For this review, take the finished solid that the model builds, in its own axes (mm). Face numbers are marked on the shaded views. Give positions to 0.01 mm unless a question says otherwise; leave off trailing zeros. Order: outer loops, then holes, each group sorted by start corner. A loop starts at its lowest first (then second) coordinate and runs counter-clockwise, first axis right, second up.
from build123d import *

# Parameters (mm, degrees)
ESQUISSE1_R        = 5.5
BOSS_EXTRU_1_DEPTH = 5
ESQUISSE3_W        = 10
ESQUISSE3_H        = 54.25
ESQUISSE3_H_2      = 42.75
ESQUISSE3_W_2      = 33
ESQUISSE3_H_3      = 10
BOSS_EXTRU_3_DEPTH = 6
D_POUILLE2_ANGLE   = 10
BOSS_EXTRU_4_DEPTH = 10
CHANFREIN1_SIZE    = 5


with BuildPart() as part:
    # Esquisse1 → Boss.-Extru.1 (new body)
    with BuildSketch(Plane.XY):
        Polygon((-22.5, 135.232443508), (22.5, 135.232443508), (70, -9.767556492), (70, -54.767556492), (-70, -54.767556492), (-70, -9.767556492), align=None)
        with Locations((0, 120.232443508)):
            Circle(ESQUISSE1_R, mode=Mode.SUBTRACT)
        with Locations((0, 43.982443508)):
            Circle(ESQUISSE1_R, mode=Mode.SUBTRACT)
        with Locations((0, -32.267556492)):
            Circle(ESQUISSE1_R, mode=Mode.SUBTRACT)
        with Locations((-55, -32.267556492)):
            Circle(ESQUISSE1_R, mode=Mode.SUBTRACT)
        with Locations((55, -32.267556492)):
            Circle(ESQUISSE1_R, mode=Mode.SUBTRACT)
    extrude(amount=BOSS_EXTRU_1_DEPTH)

    # Esquisse3 → Boss.-Extru.3 (add)
    with BuildSketch(Plane.XY.offset(5)):
        with Locations((0, 82.107443508)):
            Rectangle(ESQUISSE3_W, ESQUISSE3_H)
        with Locations((0, 11.607443508)):
            Rectangle(ESQUISSE3_W, ESQUISSE3_H_2)
        with Locations((-27.5, -32.267556492)):
            Rectangle(ESQUISSE3_W_2, ESQUISSE3_H_3)
        with Locations((27.5, -32.267556492)):
            Rectangle(ESQUISSE3_W_2, ESQUISSE3_H_3)
    extrude(amount=BOSS_EXTRU_3_DEPTH)

    # Dépouille2
    d_pouille2_faces = [part.faces().sort_by_distance(p)[0] for p in [
        (0, 32.982443508, 8),
        (-27.5, -27.267556492, 8),
        (27.5, -27.267556492, 8),
        (0, 109.232443508, 8),
        (-11, -32.267556492, 8),
        (44, -32.267556492, 8),
        (5, 82.107443508, 8),
        (5, 11.607443508, 8),
        (-5, 82.107443508, 8),
        (0, 54.982443508, 8),
        (-5, 11.607443508, 8),
        (11, -32.267556492, 8),
        (27.5, -37.267556492, 8),
        (0, -9.767556492, 8),
        (-44, -32.267556492, 8),
        (-27.5, -37.267556492, 8),
    ]]
    draft(d_pouille2_faces, Plane.XY.offset(5), D_POUILLE2_ANGLE)

    # Esquisse4 → Boss.-Extru.4 (add)
    with BuildSketch(Plane.XY.offset(5)):
        Polygon((-22.75, 134.469285613), (-22.75, -9.517556492), (-69.918103448, -9.517556492), align=None)
        Polygon((22.75, -9.517556492), (69.918103448, -9.517556492), (22.75, 134.469285613), align=None)
    extrude(amount=BOSS_EXTRU_4_DEPTH)

    # Chanfrein1
    chanfrein1_edges = [part.edges().sort_by_distance(p)[0] for p in [
        (-22.75, -9.517556492, 10),
        (22.75, -9.517556492, 10),
    ]]
    chamfer(chanfrein1_edges, length=CHANFREIN1_SIZE)


solid = part.part
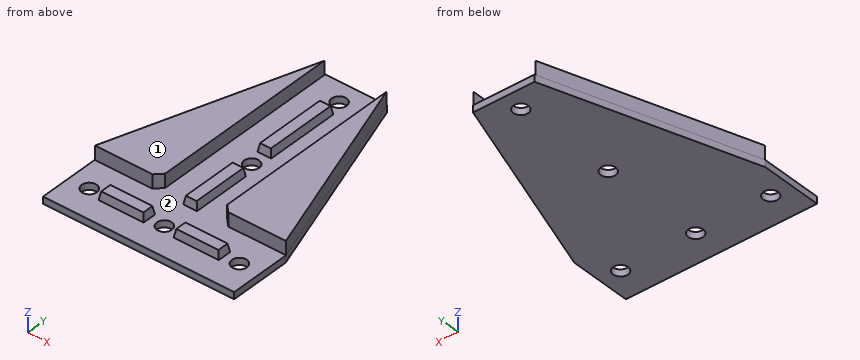
1) Draft analysis for pull direction X (two halves, no side actions). For the marked faces 1 and 2, state which applies: +X half, -X half, draft (parallel to the pull), parting line (faces both ways), or undercut.
Answer sheet:
face 1: draft
face 2: undercut
2) To check wall thickness, follow line 1 (Y direction, x = 0, z = 1.3); line 2 (X direction, y = 6, z = 6.5); line 3 (X direction, y = 80, z = 10). State the ranges of each line that lie inside material, in increasing order.
Answer sheet:
line 1: y = -54.77 to -37.77, -26.77 to 38.48, 49.48 to 114.73, 125.73 to 135.23
line 2: x = -64.83 to -22.75, -4.74 to 4.74, 22.75 to 64.83
line 3: x = -40.59 to -22.75, -4.12 to 4.12, 22.75 to 40.59
3) We need section A-A on x = 0. Give the boundary of the cut face in (y, z), then the cut area to 3 significant figures.
Answer sheet:
outline: (-54.77, 0) - (-37.77, 0) - (-37.77, 5) - (-54.77, 5) - close; (-26.77, 0) - (38.48, 0) - (38.48, 5) - (32.98, 5) - (31.92, 11) - (-8.71, 11) - (-9.77, 5) - (-26.77, 5) - close; (49.48, 0) - (114.73, 0) - (114.73, 5) - (109.23, 5) - (108.17, 11) - (56.04, 11) - (54.98, 5) - (49.48, 5) - close; (125.73, 0) - (135.23, 0) - (135.23, 5) - (125.73, 5) - close
area: 1,350 mm2
4) We need section C-C on y = 12. Give the boundary of the cut face in (x, z), then the cut area to 3 significant figures.
Answer sheet:
outline: (-62.87, 0) - (62.87, 0) - (62.87, 15) - (22.75, 15) - (22.75, 5) - (5, 5) - (3.94, 11) - (-3.94, 11) - (-5, 5) - (-22.75, 5) - (-22.75, 15) - (-62.87, 15) - close
area: 1,480 mm2
5) We need section B-B on x = -55. Give the boundary of the cut face in (y, z).
Answer sheet:
outline: (-54.77, 0) - (-37.77, 0) - (-37.77, 5) - (-54.77, 5) - close; (-26.77, 0) - (36.02, 0) - (36.02, 15) - (-9.52, 15) - (-9.52, 5) - (-26.77, 5) - close
6) We need section D-D on x = 18.5. Give the boundary of the cut face in (y, z).
Answer sheet:
outline: (-54.77, 0) - (135.23, 0) - (135.23, 5) - (-27.27, 5) - (-28.33, 11) - (-36.21, 11) - (-37.27, 5) - (-54.77, 5) - close
7) Clearance check with flat-ended pins moving along their axes: pin 1 (2.5 mm diameter, centred on x = -28, y = -32.5, fed in from +Z); pin 2 (12.5 mm diameter, centred on x = 55, y = -32.27, fed in from +Z); pin 3 (3 mm diameter, centred on y = 32.5, z = 9, fed in from -X). State where each tip first meets the part, or that it passes through.
Answer sheet:
pin 1: stops at z = 11
pin 2: stops at z = 5
pin 3: stops at x = -56.65
